Could you check a few things on this model? Use its own coordinates, in mm. A direction names the side the tool comes from. Round coordinates to 2 decimals unless told otherwise and drop trailing zeros. Order: outer loops, then holes, each group sorted by start corner. A loop starts at its lowest first (then second) coordinate and runs counter-clockwise, first axis right, second up. Notation, with made-up numbers: (42.5, -39) -> (87.5, -39) arc R22 cw to (87.5, -3) -> close; hole circle Ø9 at (16.25, 53). An arc over 180 degrees is marked (long way). Put each result on its own line as item: value. Start each with the question number.
from build123d import *

# Parameters (mm, degrees)
F0_R      = 45.72
F2_DEPTH  = 114.3
F1_R      = 36.83
F3_DEPTH  = 114.3
F4_W      = 90.153438
F4_H      = 12.7
F5_DEPTH  = 5.08
F6_W      = 12.7
F6_H      = 90.641294
F7_DEPTH  = 5.08
F8_W      = 11.431906
F8_H      = 43.256522
F9_DEPTH  = 21.59
F11_DEPTH = 50.8
F12_W     = 27.94
F12_H     = 31.50979
F13_DEPTH = 55.88


with BuildPart() as f2:
    # F0 (on Top) → F2 (new body)
    with BuildSketch(Plane.XY):
        Circle(F0_R)
    extrude(amount=F2_DEPTH)

    # F1 (on Top) → F3 (cut)
    with BuildSketch(Plane.XY):
        Circle(F1_R)
    extrude(amount=F3_DEPTH, mode=Mode.SUBTRACT)

    # F4 (on Top) → F5 (join)
    with BuildSketch(Plane.XY):
        with Locations((0, -1.292501)):
            Rectangle(F4_W, F4_H)
    extrude(amount=F5_DEPTH)

    # F6 (on Top) → F7 (join)
    with BuildSketch(Plane.XY):
        with Locations((0.320298, 0)):
            Rectangle(F6_W, F6_H)
    extrude(amount=F7_DEPTH)

    # F8 (on Right) → F9 (join, symmetric)
    with BuildSketch(Plane.YZ):
        Polygon((79.057269, 111.757322), (40.957269, 111.757322), (40.957269, 102.859358), (67.625363, 102.859358), (79.057269, 102.859358), align=None)
        with Locations((73.341316, 81.231097)):
            Rectangle(F8_W, F8_H)
    extrude(amount=F9_DEPTH, both=True)

    # F10 (on Top) → F11 (join)
    with BuildSketch(Plane.XY):
        with BuildLine():
            Line((-13.038913, 40.473972), (15.744843, 40.473972))
            Line((15.744843, 40.473972), (15.744843, 58.045961))
            Line((15.744843, 58.045961), (12.391999, 58.045961))
            ThreePointArc((12.391999, 58.045961), (1.352965, 47.006926), (-9.68607, 58.045961))
            Line((-9.68607, 58.045961), (-13.038913, 58.045961))
            Line((-13.038913, 58.045961), (-13.038913, 40.473972))
        make_face()
    extrude(amount=F11_DEPTH)

    # F12 (on face) → F13 (cut)
    with BuildSketch(Plane.XY.offset(111.757322)):
        with Locations((0.096068, 63.302374)):
            Rectangle(F12_W, F12_H)
    extrude(amount=-F13_DEPTH, mode=Mode.SUBTRACT)


solid = f2.part
1. For pin 1 Ø4.5 at (y, z) = (50.5, 38) entering from +X; pin 2 Ø3 at (x, z) = (36.5, 55) entering from +Y; pin 3 Ø3 at (x, z) = (12.5, 91.5) entering from +Y, each with a flat end and sliding along its axis, tell me the tip position at first contact or that it passes through.
2. If we section it at B-B, the plane z = 13: Please give me the cut outline in (x, y).
3. I need wall thicknesses on L1, parallel to X at y = 0, z = 45; L2, parallel to Y at x = 1, z = 13. Which ranges of each line are inside material? Lowest first, please.
4. If we section it at D-D, the plane x = -26: Please give me the cut outline in (y, z).
5. If we section it at C-C, the plane y = -22.5: Please give me the cut outline in (x, z).
6. If we section it at A-A, the plane z = 74: Please give me the cut outline in (x, y), then the cut area to 3 significant figures.
7. Which directions (+Z, -Z, +X, -X, +Y, -Y) give clear straight access to the entire face, cutting with the end or side of a thin tool? Please do faces 1 (the face through (-13.874, 70, 92)), 2 (the face through (-13.039, 51, 25)), 3 (the face through (-18, 73, 59.603)), 4 (the face through (-6.03, 20, 3)), 5 (the face through (-18, 67.625, 81)).
8. Thinking about a two-plate mould opening in Y: for faces 6 (the face through (21.59, 68, 92)), 7 (the face through (18, 79.057, 85)), 8 (the face through (-29.227, -22.41, 56.35)), which applies, +Y half, -Y half, draft (parallel to the pull), parting line (faces both ways), or undercut?
Results below:
1. pin 1: x = 15.74
1. pin 2: y = 29.42
1. pin 3: y = 44.38
2. outline: (-13.04, 43.82) arc R45.72 ccw (long way) to (15.74, 42.92) -> (15.74, 58.05) -> (12.39, 58.05) arc R11.04 cw to (-9.69, 58.05) -> (-13.04, 58.05) -> close; hole circle Ø73.66 at (0, 0)
3. L1: -45.72 to -36.83, 36.83 to 45.72
3. L2: -45.71 to -36.82, 36.82 to 47.01
4. outline: (-37.61, 0) -> (-26.09, 0) -> (-26.09, 114.3) -> (-37.61, 114.3) -> close; (-7.64, 0) -> (5.06, 0) -> (5.06, 5.08) -> (-7.64, 5.08) -> close; (26.09, 0) -> (37.61, 0) -> (37.61, 114.3) -> (26.09, 114.3) -> close
5. outline: (-39.8, 0) -> (-29.16, 0) -> (-29.16, 114.3) -> (-39.8, 114.3) -> close; (-6.03, 0) -> (6.67, 0) -> (6.67, 5.08) -> (-6.03, 5.08) -> close; (29.16, 0) -> (39.8, 0) -> (39.8, 114.3) -> (29.16, 114.3) -> close
6. outline: circle Ø91.44 at (0, 0); (-21.59, 67.63) -> (-13.87, 67.63) -> (-13.87, 79.06) -> (-21.59, 79.06) -> close; (14.07, 67.63) -> (21.59, 67.63) -> (21.59, 79.06) -> (14.07, 79.06) -> close; hole circle Ø73.66 at (0, 0)
6. area: 2,480 mm2
7. face 1: +Z, -Z, +Y
7. face 2: -Z, -X, +Y
7. face 3: -Z, +X, -X, +Y
7. face 4: +Z, -Z
7. face 5: -Z, +X, -X
8. face 6: draft
8. face 7: +Y half
8. face 8: undercut
